Source: CAD feature listing. Evaluate the final solid. Frame: model axes, mm. A direction names the side the tool comes from. Give positions to 0.01 mm unless a question says otherwise; leave off trailing zeros. Write each loop counter-clockwise with the first axis right and the second up, starting at its lowest first coordinate (ties: lowest second). Pieces come first, ordered by that corner, then holes. Notation, with made-up numbers: M 37.25,20.25 L 78.25,20.25 A25 ccw 78.25,52.25 Z; hole C 58.5,18 d11. An arc over 180 degrees is marked long. Answer as a JSON object with one key per item and string values. Group by question number.
```python
from build123d import *

# Parameters (mm, degrees)
SKETCH1_W           = 54
SKETCH1_H           = 54
SKETCH1_R           = 4.25
BOSS_EXTRUDE1_DEPTH = 7
FILLET2_R           = 6.5
SKETCH2_R           = 22
CUT_EXTRUDE1_DEPTH  = 1.6
SKETCH3_R           = 19.2
CUT_EXTRUDE2_DEPTH  = 3.2


with BuildPart() as part:
    # Sketch1 → Boss-Extrude1 (new body)
    with BuildSketch(Plane(origin=(0, 0, 0), x_dir=(1, 0, 0), z_dir=(0, 1, 0))):
        Rectangle(SKETCH1_W, SKETCH1_H)
        with Locations(Location((-20.329319959, 20.329319959, 0), (0, 0, 270))):
            Circle(SKETCH1_R, mode=Mode.SUBTRACT)
        with Locations(Location((20.329319959, -20.329319959, 0), (0, 0, 90))):
            Circle(SKETCH1_R, mode=Mode.SUBTRACT)
        with Locations(Location((-20.329319959, -20.329319959, 0), (0, 0, 270))):
            Circle(SKETCH1_R, mode=Mode.SUBTRACT)
        with Locations(Location((20.329319959, 20.329319959, 0), (0, 0, 90))):
            Circle(SKETCH1_R, mode=Mode.SUBTRACT)
    extrude(amount=BOSS_EXTRUDE1_DEPTH)

    # Fillet2
    fillet2_edges = [part.edges().sort_by_distance(p)[0] for p in [
        (27, 3.5, 27),
        (-27, 3.5, 27),
        (-27, 3.5, -27),
        (27, 3.5, -27),
    ]]
    fillet(fillet2_edges, radius=FILLET2_R)

    # Sketch2 → Cut-Extrude1 (cut)
    with BuildSketch(Plane(origin=(0, 7, 0), x_dir=(1, 0, 0), z_dir=(0, 1, 0))):
        with Locations(Location((0, 0, 0), (0, 0, 270))):
            Circle(SKETCH2_R)
    extrude(amount=-CUT_EXTRUDE1_DEPTH, mode=Mode.SUBTRACT)

    # Sketch3 → Cut-Extrude2 (cut)
    with BuildSketch(Plane(origin=(0, 5.4, 0), x_dir=(1, 0, 0), z_dir=(0, 1, 0))):
        with Locations(Location((0, 0, 0), (0, 0, 270))):
            Circle(SKETCH3_R)
    extrude(amount=-CUT_EXTRUDE2_DEPTH, mode=Mode.SUBTRACT)


solid = part.part
```
(1) Pull-direction query (Z, two-part tool) for faces 3 (the cylindrical face through (-25.146, 3.549, 25.045)), 4 (the cylindrical face through (25.045, 3.549, -25.146)), 5 (the cylindrical face through (22.92, 3.45, 23.7)); classes: pulls with the +Z half, pulls with the -Z half, needs draft (parallel to the pull), parting line crosses it, or undercut.
(2) Section A-A, the plane x = 0. Return loops of the section in (y, z).
(3) Section B-B, the plane x = -18. Return loops of the section in (y, z), plus the area to 3 significant figures.
(4) Contact query for a flat-ended pin moving along its axis: pin 1 Ø11.5 at (x, z) = (-7.5, -6.5) entering from +Y. Output: stop coordinate, or through.
(5) Access query for faces 1 (the cylindrical face through (-21.477, 6.211, -4.769)), 2 (the flat face through (-27, 3, 0)). Directions: +Z, -Z, +X, -X, +Y, -Y. A direction counts if a zero-diameter tool reaches every point of the face in a straight line with its end or side. Return the directions, or none.
(6) Ray query, L1, parallel to Z at x = -20, y = 2; L2, parallel to Z at x = -17, y = 5. Return the intervals inside material, ascending. Write a range as [from, to].
(7) Section C-C, the plane z = 0. Return loops of the section in (x, y), plus the area to 3 significant figures.
Reported:
{
 "1": {"face 3": "pulls with the +Z half", "face 4": "pulls with the -Z half", "face 5": "undercut"},
 "2": {"outline": "M 0,-27 L 7,-27 L 7,-22 L 5.4,-22 L 5.4,-19.2 L 2.2,-19.2 L 2.2,19.2 L 5.4,19.2 L 5.4,22 L 7,22 L 7,27 L 0,27 Z"},
 "3": {"outline": "M 0,-27 L 7,-27 L 7,-23.88 L 0,-23.88 Z; M 0,-16.77 L 7,-16.77 L 7,-12.65 L 5.4,-12.65 L 5.4,-6.68 L 2.2,-6.68 L 2.2,6.68 L 5.4,6.68 L 5.4,12.65 L 7,12.65 L 7,16.77 L 0,16.77 Z; M 0,23.88 L 7,23.88 L 7,27 L 0,27 Z", "area": "195 mm2"},
 "4": {"pin 1": "stops at y = 2.2"},
 "5": {"face 1": "+Y", "face 2": "+Z, -Z, -X, +Y, -Y"},
 "6": {"L1": "z = [-27, -24.57], [-16.09, 16.09], [24.57, 27]", "L2": "z = [-27, -22.97], [-17.69, -8.92], [8.92, 17.69], [22.97, 27]"},
 "7": {"outline": "M -27,0 L 27,0 L 27,7 L 22,7 L 22,5.4 L 19.2,5.4 L 19.2,2.2 L -19.2,2.2 L -19.2,5.4 L -22,5.4 L -22,7 L -27,7 Z", "area": "185 mm2"}
}
